from build123d import *

# Parameters (mm, degrees)
CROQUIS1_R                = 3
SALIENTE_EXTRUIR1_DEPTH   = 4
SALIENTE_EXTRUIR1_2_DEPTH = 4
CROQUIS2_W                = 90
CROQUIS2_H                = 6
SALIENTE_EXTRUIR2_DEPTH   = 4
CROQUIS4_W                = 46
CROQUIS4_H                = 13
SALIENTE_EXTRUIR3_DEPTH   = 6
CROQUIS5_W                = 38
CROQUIS5_H                = 13
CORTAR_EXTRUIR1_DEPTH     = 95.09569597
CROQUIS6_W                = 8
CROQUIS6_H                = 9
SALIENTE_EXTRUIR4_DEPTH   = 3
CROQUIS7_W                = 3.5
CROQUIS7_H                = 8.2
CORTAR_EXTRUIR2_DEPTH     = 96.754895436
CHAFL_N1_SIZE             = 3
REDONDEO1_R               = 1
CROQUIS8_R                = 1.75
CORTAR_EXTRUIR3_DEPTH     = 97.612628574
SALIENTE_EXTRUIR5_DEPTH   = 4
CROQUIS10_R               = 2
CORTAR_EXTRUIR4_DEPTH     = 97.586748573
CHAFL_N2_SIZE             = 0.5


with BuildPart() as part:
    # Croquis1 → Saliente-Extruir1 (new body)
    with BuildSketch(Plane.XY):
        Circle(CROQUIS1_R)
    extrude(amount=SALIENTE_EXTRUIR1_DEPTH)



with BuildPart() as body_2:
    # Croquis1 → Saliente-Extruir1 2 (new body)
    with BuildSketch(Plane.XY):
        with Locations((90, 0)):
            Circle(CROQUIS1_R)
    extrude(amount=SALIENTE_EXTRUIR1_2_DEPTH)


with BuildPart() as part_1:
    add(part.part)

    add(body_2.part)  # Saliente-Extruir2 merges body 2
    # Croquis2 → Saliente-Extruir2 (add)
    with BuildSketch(Plane.XY):
        with Locations((45, 0)):
            Rectangle(CROQUIS2_W, CROQUIS2_H)
    extrude(amount=SALIENTE_EXTRUIR2_DEPTH)

    # Croquis4 → Saliente-Extruir3 (add)
    with BuildSketch(Plane(origin=(0, 3, 0), x_dir=(1, 0, 0), z_dir=(0, 1, 0))):
        with Locations((45, 6.5)):
            Rectangle(CROQUIS4_W, CROQUIS4_H)
    extrude(amount=-SALIENTE_EXTRUIR3_DEPTH)

    # Croquis5 → Cortar-Extruir1 (cut, through all)
    with BuildSketch(Plane(origin=(0, 3, 0), x_dir=(1, 0, 0), z_dir=(0, 1, 0))):
        with Locations((45, 2.5)):
            Rectangle(CROQUIS5_W, CROQUIS5_H)
    extrude(amount=-CORTAR_EXTRUIR1_DEPTH, mode=Mode.SUBTRACT)

    # Croquis6 → Saliente-Extruir4 (add, symmetric)
    with BuildSketch(Plane(origin=(0, 0, 0), x_dir=(1, 0, 0), z_dir=(0, 1, 0))):
        with Locations((40, 17.5)):
            Rectangle(CROQUIS6_W, CROQUIS6_H)
    extrude(amount=SALIENTE_EXTRUIR4_DEPTH, both=True)

    # Croquis7 → Cortar-Extruir2 (cut, through all)
    with BuildSketch(Plane(origin=(0, 3, 0), x_dir=(1, 0, 0), z_dir=(0, 1, 0))):
        with Locations((40, 17.1)):
            Rectangle(CROQUIS7_W, CROQUIS7_H)
    extrude(amount=-CORTAR_EXTRUIR2_DEPTH, mode=Mode.SUBTRACT)

    # Chaflán1
    chafl_n1_edges = [part_1.edges().sort_by_distance(p)[0] for p in [
        (22, 0, 0),
        (68, 0, 0),
        (26, 0, -9),
        (64, 0, -9),
        (36, 0, -13),
        (44, 0, -13),
    ]]
    chamfer(chafl_n1_edges, length=CHAFL_N1_SIZE)

    # Redondeo1
    redondeo1_edges = [part_1.edges().sort_by_distance(p)[0] for p in [
        (22, 0, -13),
        (68, 0, -13),
        (26, 0, 4),
        (64, 0, 4),
        (36, 0, -22),
        (44, 0, -22),
        (38.25, 0, -13),
        (38.25, 0, -21.2),
        (41.75, 0, -21.2),
        (41.75, 0, -13),
    ]]
    fillet(redondeo1_edges, radius=REDONDEO1_R)

    # Croquis8 → Cortar-Extruir3 (cut, through all)
    with BuildSketch(Plane.XY.offset(4)):
        Circle(CROQUIS8_R)
        with Locations((90, 0)):
            Circle(CROQUIS8_R)
    extrude(amount=-CORTAR_EXTRUIR3_DEPTH, mode=Mode.SUBTRACT)

    # Croquis9 → Saliente-Extruir5 (add)
    with BuildSketch(Plane.XY.offset(4)):
        with BuildLine():
            Line((-1, 3), (0, 3))
            Line((0, 3), (0, 2.5))
            ThreePointArc((0, 2.5), (-2.5, 0), (0, -2.5))
            Line((0, -2.5), (0, -3))
            Line((0, -3), (-1, -3))
            ThreePointArc((-1, -3), (-4, 0), (-1, 3))
        make_face()
    saliente_extruir5 = extrude(amount=-SALIENTE_EXTRUIR5_DEPTH)

    # Simetría1: Saliente-Extruir5 across plane
    add(saliente_extruir5.mirror(Plane(origin=(45, 0, 0), x_dir=(0, 0, 1), z_dir=(1, 0, 0))))

    # Croquis10 → Cortar-Extruir4 (cut, through all)
    with BuildSketch(Plane(origin=(0, 0, 0), x_dir=(-1, 0, 0), z_dir=(0, 0, -1))):
        Circle(CROQUIS10_R)
        with Locations((-90, 0)):
            Circle(CROQUIS10_R)
    extrude(amount=-CORTAR_EXTRUIR4_DEPTH, mode=Mode.SUBTRACT)

    # Chaflán2
    # the kernel refuses this chamfer: 0.5 mm, written as the material it takes off along each edge
    with BuildSketch(Plane(origin=(63.714158506, 3, 4), x_dir=(0, 0.027495876610586487, -0.9996219169112968), z_dir=(1, 0, 0)), Plane(origin=(-1, -3, 4), x_dir=(0, 0.9996219169112968, 0.027495876610585623), z_dir=(1, 0, 0)), Plane(origin=(-1, 3, 4), x_dir=(0, 0.027495876610590796, -0.9996219169112965), z_dir=(1, 0, 0)), Plane(origin=(63.714158506, -3, 4), x_dir=(0, 0.9996219169112968, 0.027495876610585623), z_dir=(1, 0, 0))) as chafl_n2_piece_1:
        Polygon((CHAFL_N2_SIZE * 0.999621916911, -CHAFL_N2_SIZE * 0.0274958766106), (-CHAFL_N2_SIZE * 0.0274958766106, -CHAFL_N2_SIZE * 0.999621916911), (0, 0), align=None)
    extrude(amount=27.285841494, mode=Mode.SUBTRACT)
    with BuildSketch(Plane(origin=(-1, 0, 0), x_dir=(0, -1, 0), z_dir=(1, 0, 0))) as chafl_n2_piece_2:
        Polygon((3, -CHAFL_N2_SIZE), (3 - CHAFL_N2_SIZE, 0), (3, 0), align=None)
    revolve(axis=Axis((-1, 0, 0), (0, 0, -1)), revolution_arc=180, mode=Mode.SUBTRACT)
    with BuildSketch(Plane(origin=(-1, 0, 4), x_dir=(0, -1, 0), z_dir=(1, 0, 0))) as chafl_n2_piece_3:
        Polygon((3 - CHAFL_N2_SIZE, 0), (3, CHAFL_N2_SIZE), (3, 0), align=None)
    revolve(axis=Axis((-1, 0, 4), (0, 0, -1)), revolution_arc=180, mode=Mode.SUBTRACT)
    with BuildSketch(Plane(origin=(91, 0, 4), x_dir=(0, -1, 0), z_dir=(-1, 0, 0))) as chafl_n2_piece_4:
        Polygon((3, -CHAFL_N2_SIZE), (3 - CHAFL_N2_SIZE, 0), (3, 0), align=None)
    revolve(axis=Axis((91, 0, 4), (0, 0, 1)), revolution_arc=180, mode=Mode.SUBTRACT)
    with BuildSketch(Plane(origin=(91, 0, 0), x_dir=(0, -1, 0), z_dir=(-1, 0, 0))) as chafl_n2_piece_5:
        Polygon((3 - CHAFL_N2_SIZE, 0), (3, CHAFL_N2_SIZE), (3, 0), align=None)
    revolve(axis=Axis((91, 0, 0), (0, 0, 1)), revolution_arc=180, mode=Mode.SUBTRACT)
    with BuildSketch(Plane(origin=(91, -3, 0), x_dir=(0, 0.9996219169112968, -0.027495876610586365), z_dir=(-1, 0, 0))) as chafl_n2_piece_6_section:
        Polygon((CHAFL_N2_SIZE * 0.999621916911, -CHAFL_N2_SIZE * 0.0274958766106), (-CHAFL_N2_SIZE * 0.0274958766106, -CHAFL_N2_SIZE * 0.999621916911), (0, 0), align=None)
    chafl_n2_piece_6 = extrude(amount=21.285841494, mode=Mode.PRIVATE)
    chafl_n2_piece_6 = split(chafl_n2_piece_6, bisect_by=Plane(origin=(80.80759364, -2.786891573, 9.80759364), z_dir=(0.7071067811865476, 0, -0.7071067811865476)), keep=Keep.TOP, mode=Mode.PRIVATE)
    add(chafl_n2_piece_6, mode=Mode.SUBTRACT)
    with BuildSketch(Plane(origin=(20.285841494, -3, 0), x_dir=(0, 0.9996219169112968, -0.027495876610586365), z_dir=(-1, 0, 0))) as chafl_n2_piece_7_section:
        Polygon((CHAFL_N2_SIZE * 0.999621916911, -CHAFL_N2_SIZE * 0.0274958766106), (-CHAFL_N2_SIZE * 0.0274958766106, -CHAFL_N2_SIZE * 0.999621916911), (0, 0), align=None)
    chafl_n2_piece_7 = extrude(amount=21.285841494, mode=Mode.PRIVATE)
    chafl_n2_piece_7 = split(chafl_n2_piece_7, bisect_by=Plane(origin=(14.099970333, -2.8351922, 4.900029667), z_dir=(-0.7071067811865476, 0, -0.7071067811865476)), keep=Keep.TOP, mode=Mode.PRIVATE)
    add(chafl_n2_piece_7, mode=Mode.SUBTRACT)
    with BuildSketch(Plane(origin=(20.285841494, 3, 0), x_dir=(0, 0.027495876610586494, 0.9996219169112968), z_dir=(-1, 0, 0))) as chafl_n2_piece_8_section:
        Polygon((CHAFL_N2_SIZE * 0.999621916911, -CHAFL_N2_SIZE * 0.0274958766106), (-CHAFL_N2_SIZE * 0.0274958766106, -CHAFL_N2_SIZE * 0.999621916911), (0, 0), align=None)
    chafl_n2_piece_8 = extrude(amount=21.285841494, mode=Mode.PRIVATE)
    chafl_n2_piece_8 = split(chafl_n2_piece_8, bisect_by=Plane(origin=(14.099970416, 2.835192201, 4.900029584), z_dir=(-0.7071067811865476, 0, -0.7071067811865476)), keep=Keep.TOP, mode=Mode.PRIVATE)
    add(chafl_n2_piece_8, mode=Mode.SUBTRACT)
    with BuildSketch(Plane(origin=(91, 3, 0), x_dir=(0, 0.027495876610590803, 0.9996219169112965), z_dir=(-1, 0, 0))) as chafl_n2_piece_9_section:
        Polygon((CHAFL_N2_SIZE * 0.999621916911, -CHAFL_N2_SIZE * 0.0274958766106), (-CHAFL_N2_SIZE * 0.0274958766106, -CHAFL_N2_SIZE * 0.999621916911), (0, 0), align=None)
    chafl_n2_piece_9 = extrude(amount=21.285841494, mode=Mode.PRIVATE)
    chafl_n2_piece_9 = split(chafl_n2_piece_9, bisect_by=Plane(origin=(75.900029584, 2.835192201, 4.900029584), z_dir=(0.7071067811865476, 0, -0.7071067811865476)), keep=Keep.TOP, mode=Mode.PRIVATE)
    add(chafl_n2_piece_9, mode=Mode.SUBTRACT)


solid = part_1.part
Work out the finished part from the listing and answer in its coordinate system (mm). A direction names the side the tool comes from. Give positions to 0.01 mm unless a question says otherwise; leave off trailing zeros. Order: outer loops, then holes, each group sorted by start corner. A loop starts at its lowest first (then second) coordinate and runs counter-clockwise, first axis right, second up. Notation, with made-up numbers: (69, 13.25) -> (79, 13.25) arc R8 cw to (79, 19.25) -> close; hole circle Ø5 at (-34, -4). An arc over 180 degrees is marked (long way). Answer as a JSON object with one key per item and string values. Group by question number.
1. The mould has two halves that part along Y. Classify faces 1 (the cylindrical face through (88.092, 0.601, 1.972)), 2 (the flat face through (8, 0, 0)), 3 (the flat face through (45.2, 3, -9.2)), 4 (the flat face through (44.8, -3, -9.2)): released by +Y, released by -Y, zero draft, split by the parting line, or undercut.
2. Section C-C on z = -1.25 is taken. Determine the outline of the cut face in (x, y), plus the area to 3 significant figures.
3. Flat-ended cylindrical pins translate along their axes: pin 1 Ø3 at (y, z) = (0.5, -3.5) entering from +X; pin 2 Ø3 at (y, z) = (-1, -9.5) entering from +X; pin 3 Ø3 at (y, z) = (-0.5, -9) entering from -X; pin 4 Ø8 at (x, z) = (65.5, -14.5) entering from +Y. Find the tip coordinate at first contact, or state that the pin passes through.
4. A tool of negligible diameter and unlimited length cuts with its end or side. For faces 5 (the flat face through (64, 0, -1)), 6 (the cylindrical face through (94, 0, 2)), 7 (the conical face through (93.635, -0.058, 3.865)), 8 (the flat face through (22, 0, -7)), 9 (the flat face through (57, 0, -13)), from which of +Z, -Z, +X, -X, +Y, -Y can it reach the whole face along a straight path? Write none if from no direction.
5. Section B-B on x = 90 is taken. Determine the outline of the cut face in (y, z), plus the area to 3 significant figures.
6. Section A-A on z = -18 is taken. Determine the outline of the cut face in (x, y).
7. Section D-D on x = 20.5 is taken. Determine the outline of the cut face in (y, z).
8. Consider line 1 along Y through (x, z) = (0, 1.2); line 2 along X through (y, z) = (-0.5, 2.75); line 3 along X through (y, z) = (0.25, -10.75). Determine where each line is inside the solid, lowest interval first. Write a range as [from, to].
Result sheet:
{
 "1": {"face 1": "undercut", "face 2": "zero draft", "face 3": "released by +Y", "face 4": "released by -Y"},
 "2": {"outline": "(20.25, -3) -> (26, -3) -> (26, 3) -> (20.25, 3) -> close; (64, -3) -> (69.75, -3) -> (69.75, 3) -> (64, 3) -> close", "area": "69.0 mm^2"},
 "3": {"pin 1": "stops at x = 69", "pin 2": "stops at x = 68", "pin 3": "stops at x = 22", "pin 4": "stops at y = 3"},
 "4": {"face 5": "+Z, +Y, -Y", "face 6": "+Z, -Z, +X", "face 7": "+Z, +X", "face 8": "-Z, -X, +Y, -Y", "face 9": "-Z, +X, +Y, -Y"},
 "5": {"outline": "(-3, 0.5) -> (-2.5, 0) -> (-2, 0) -> (-2, 4) -> (-2.5, 4) -> (-3, 3.5) -> close; (2, 0) -> (2.5, 0) -> (3, 0.5) -> (3, 3.5) -> (2.5, 4) -> (2, 4) -> close", "area": "7.50 mm^2"},
 "6": {"outline": "(36, -3) -> (38.25, -3) -> (38.25, 3) -> (36, 3) -> close; (41.75, -3) -> (44, -3) -> (44, 3) -> (41.75, 3) -> close"},
 "7": {"outline": "(-3, -1.5) -> (3, -1.5) -> (3, 3.5) -> (2.5, 4) -> (-2.5, 4) -> (-3, 3.5) -> close"},
 "8": {"line 1": "y = [-3, -2], [2, 3]", "line 2": "x = [-3.96, -1.94], [1.94, 26], [64, 88.06], [91.94, 93.96]", "line 3": "x = [22, 68]"}
}
